The model under review builds one solid part; all positions refer to its coordinate system, in mm. Face numbers are marked on the shaded views. A direction names the side the tool comes from. Coordinates: 2 decimals unless noted, no trailing zeros. One line per item, written item: value.
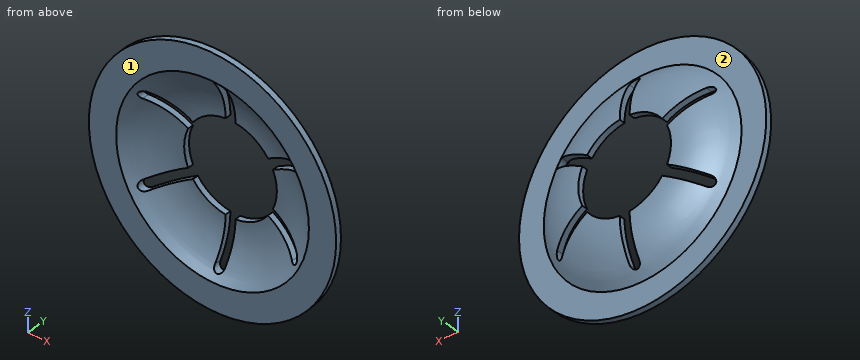
```python
from build123d import *

# Parameters (mm, degrees)
CUT_EXTRUDE1_DEPTH = 12.456002809
CIRPATTERN1_COUNT  = 6


with BuildPart() as part:
    # Sketch2 → Revolve1 (revolve)
    with BuildSketch(Plane.XY, mode=Mode.PRIVATE) as revolve1_sk:
        with BuildLine():
            Line((-8, 0), (-6.237085417, 0))
            ThreePointArc((-6.237085417, 0), (-4.767221194, 1.048671922), (-3, 1.419))
            Line((-3, 1.419), (-3, 1.8))
            ThreePointArc((-3, 1.8), (-4.842115699, 1.431016827), (-6.4, 0.381))
            Line((-6.4, 0.381), (-8, 0.381))
            Line((-8, 0.381), (-8, 0))
        make_face()
    revolve(revolve1_sk.sketch.rotate(Axis((0, 0, 0), (0, 1, 0)), 180), axis=Axis((0, 0, 0), (0, 1, 0)))

    # Sketch3 → Cut-Extrude1 (cut, through all)
    with BuildSketch(Plane(origin=(0, 0, 0), x_dir=(1, 0, 0), z_dir=(0, 1, 0))):
        with BuildLine():
            Line((-0.3175, 5.5745), (-0.3175, 0))
            Line((-0.3175, 0), (0.3175, 0))
            Line((0.3175, 0), (0.3175, 5.5745))
            ThreePointArc((0.3175, 5.5745), (0, 5.892), (-0.3175, 5.5745))
        make_face()
    cut_extrude1 = extrude(amount=CUT_EXTRUDE1_DEPTH, mode=Mode.SUBTRACT)

    # CirPattern1: Cut-Extrude1 ×6 about axis
    cirpattern1_axis = Axis((0, 0, 0), (0, 1, 0))
    for i in range(1, CIRPATTERN1_COUNT):
        add(cut_extrude1.rotate(cirpattern1_axis, i * 360 / CIRPATTERN1_COUNT), mode=Mode.SUBTRACT)


solid = part.part
```
(1) For L1, parallel to Y at x = -7, z = 3.75; L2, parallel to X at y = 0.7, z = -3.25; L3, parallel to X at y = 0.55, z = -3.25, list the stretches that pass through material, from the lowest coordinate up.
Geometry results:
L1: y = 0 to 0.38
L2: x = -5.1 to -4.33, 4.33 to 5.1
L3: x = -5.31 to -4.59, 4.59 to 5.31
(2) We need section A-A, the plane x = 4.25. Count the separate pieces of the cut face and the enclosed holes in it, plus the area to 3 significant figures.
Geometry results:
separate pieces: 3
enclosed holes: 0
area: 5.04 mm2
(3) Insertion check: pin 1 Ø1.5 at (x, z) = (-0.5, 2.5) entering from -Y; pin 2 Ø1 at (y, z) = (1, 4) entering from +X; pin 3 Ø0.6 at (y, z) = (1, -4) entering from +X. Each pin has a flat end and moves straight along its axis. Give the tip position at first contact, or say it passes through.
Geometry results:
pin 1: stops at y = 1.41
pin 2: stops at x = 4.94
pin 3: stops at x = 4.61
(4) Tool access review of the marked faces 1 and 2: name each direction out of +Z, -Z, +X, -X, +Y, -Y from which nothing blocks a thin tool from reaching the whole face with its end or side.
Geometry results:
face 1: +Z, -Z, +X, -X, -Y
face 2: +Y
